Could you check a few things on this model? Use its own coordinates, in mm. A direction names the side the tool comes from. Coordinates: 2 decimals unless noted, no trailing zeros. Order: outer loops, then holes, each group sorted by start corner. A loop starts at its lowest first (then second) coordinate and runs counter-clockwise, first axis right, second up. Notation, with made-up numbers: (47.5, 44) - (86.5, 44) arc R14 cw to (86.5, 51) - close; hole circle Ø11 at (89.5, 71.25). An arc over 180 degrees is marked (long way). Answer as a JSON object with one key per item and string values. Group by question number.
(1) Imagine slicing it at D-D, the plane y = 19. Write out the boundary of the cut face in (x, z), and give its area (3 significant figures).
(2) Will these pins go through, and if not, where does the flat tip stop? P1, Ø8, axis at x = 50, y = -1.5, coming from the -Z side; P2, Ø3, axis at x = 42.5, y = 0, coming from the +Z side; P3, Ø1.5, axis at x = 49.5, z = 2, coming from the +Y side; P4, Ø1.5, axis at x = 49.5, z = 2, coming from the -Y side.
(3) We'd pull the mould along X, two halves only. Please class faces 3 (the flat face through (56.383, 0, 1)), 4 (the flat face through (50, -19.95, 1)), 5 (the cylindrical face through (31.8, -30.8, 1.5)): pulls with the +X half, pulls with the -X half, needs draft (parallel to the pull), parting line crosses it, or undercut.
(4) Imagine slicing it at A-A, the plane y = 0. Write out the boundary of the cut face in (x, z), and give its area (3 significant figures).
(5) Imagine slicing it at B-B, the plane x = 42.5. Write out the boundary of the cut face in (y, z), and give its area (3 significant figures).
(6) Which directions (+Z, -Z, +X, -X, +Y, -Y) give clear straight access to the entire face, cutting with the end or side of a thin tool? Please do faces 1 (the flat face through (50, 19.95, 1)), 2 (the flat face through (37, 1, 3)).
(7) Imagine slicing it at C-C, the plane z = 2.15. Write out the boundary of the cut face in (x, y) (3 decimals), and give its area (3 significant figures).
(8) Please list where these lines run through material, in increasing order: probe 1 along Y at (x, z) = (30, 1.65); probe 2 along Y at (x, z) = (42.5, 2.4); probe 3 along Y at (x, z) = (53, 1.95).
from build123d import *

# Parameters (mm, degrees)
SKETCH_1_R          = 47.75
SKETCH_1_R_2        = 32.5
SKETCH_1_R_3        = 1.9
EXTRUDE_1_DEPTH     = 3
SKETCH_2_R          = 1.9
CUT_EXTRUDE_1_DEPTH = 3
EXTRUDE_2_DEPTH     = 3
FILLET_1_R          = 3
FILLET_2_R          = 6


with BuildPart() as part:
    # 草图1 → 凸台-拉伸1 (new body)
    with BuildSketch(Plane.XY):
        Circle(SKETCH_1_R)
        Circle(SKETCH_1_R_2, mode=Mode.SUBTRACT)
        with Locations((0, 42.5)):
            Circle(SKETCH_1_R_3, mode=Mode.SUBTRACT)
        with Locations((30.0520382, 30.0520382)):
            Circle(SKETCH_1_R_3, mode=Mode.SUBTRACT)
        with Locations((42.5, 0)):
            Circle(SKETCH_1_R_3, mode=Mode.SUBTRACT)
        with Locations((30.0520382, -30.0520382)):
            Circle(SKETCH_1_R_3, mode=Mode.SUBTRACT)
        with Locations((0, -42.5)):
            Circle(SKETCH_1_R_3, mode=Mode.SUBTRACT)
        with Locations((-30.0520382, -30.0520382)):
            Circle(SKETCH_1_R_3, mode=Mode.SUBTRACT)
        with Locations((-42.5, 0)):
            Circle(SKETCH_1_R_3, mode=Mode.SUBTRACT)
        with Locations((-30.0520382, 30.0520382)):
            Circle(SKETCH_1_R_3, mode=Mode.SUBTRACT)
    extrude(amount=EXTRUDE_1_DEPTH)

    # 草图2 → 切除-拉伸1 (cut)
    # profile 1 of 2: a face of its own
    with BuildSketch(Plane(origin=(0, 0, 0), x_dir=(-1, 0, 0), z_dir=(0, 0, -1))):
        with BuildLine():
            ThreePointArc((40.6, 0), (42.5, 1.9), (44.4, 0))
            Line((44.4, 0), (47.75, 0))
            ThreePointArc((47.75, 0), (19.569412493, 43.555718278), (-31.709710772, 35.700934761))
            ThreePointArc((-31.709710772, 35.700934761), (-23.521159741, 36.955232453), (-19.021118385, 30))
            ThreePointArc((-19.021118385, 30), (-19.69088588, 26.875041473), (-21.582525806, 24.29906541))
            ThreePointArc((-21.582525806, 24.29906541), (13.319495322, 29.645253319), (32.5, 0))
            Line((32.5, 0), (40.6, 0))
        make_face()
        with Locations((0, 42.5)):
            Circle(SKETCH_2_R, mode=Mode.SUBTRACT)
        with Locations((30.0520382, 30.0520382)):
            Circle(SKETCH_2_R, mode=Mode.SUBTRACT)
    # profile 2 of 2: a face of its own
    with BuildSketch(Plane(origin=(0, 0, 0), x_dir=(-1, 0, 0), z_dir=(0, 0, -1))):
        with BuildLine():
            Line((47.75, 0), (44.4, 0))
            ThreePointArc((44.4, 0), (42.5, -1.9), (40.6, 0))
            Line((40.6, 0), (32.5, 0))
            ThreePointArc((32.5, 0), (13.319495418, -29.645253276), (-21.582525651, -24.299065549))
            ThreePointArc((-21.582525651, -24.299065549), (-19.690885837, -26.875041568), (-19.021118385, -30))
            ThreePointArc((-19.021118385, -30), (-23.521159897, -36.955232523), (-31.709711027, -35.700934534))
            ThreePointArc((-31.709711027, -35.700934534), (19.569412338, -43.555718347), (47.75, 0))
        make_face()
        with Locations((0, -42.5)):
            Circle(SKETCH_2_R, mode=Mode.SUBTRACT)
        with Locations((30.0520382, -30.0520382)):
            Circle(SKETCH_2_R, mode=Mode.SUBTRACT)
    extrude(amount=-CUT_EXTRUDE_1_DEPTH, mode=Mode.SUBTRACT)

    # 草图3 → 凸台-拉伸2 (add)
    with BuildSketch(Plane(origin=(0, 0, 0), x_dir=(-1, 0, 0), z_dir=(0, 0, -1))):
        with BuildLine():
            Line((-43.382715452, 19.95), (-56.382715452, 19.95))
            Line((-56.382715452, 19.95), (-56.382715452, 0))
            Line((-56.382715452, 0), (-47.75, 0))
            ThreePointArc((-47.75, 0), (-46.645402575, 10.211215333), (-43.382715452, 19.95))
        make_face()
        with BuildLine():
            Line((-47.75, 0), (-56.382715452, 0))
            Line((-56.382715452, 0), (-56.382715452, -19.95))
            Line((-56.382715452, -19.95), (-43.382715452, -19.95))
            ThreePointArc((-43.382715452, -19.95), (-46.645402575, -10.211215333), (-47.75, 0))
        make_face()
    extrude(amount=-EXTRUDE_2_DEPTH)

    # 圆角1
    fillet_1_edges = [part.edges().sort_by_distance(p)[0] for p in [
        (56.382715452, -19.95, 1.5),
        (56.382715452, 19.95, 1.5),
    ]]
    fillet(fillet_1_edges, radius=FILLET_1_R)

    # 圆角2
    fillet_2_edges = [part.edges().sort_by_distance(p)[0] for p in [
        (43.382715452, 19.95, 1.5),
        (43.382715452, -19.95, 1.5),
    ]]
    fillet(fillet_2_edges, radius=FILLET_2_R)


solid = part.part
Result set:
{
 "1": {"outline": "(26.37, 0) - (55.57, 0) - (55.57, 3) - (26.37, 3) - close", "area": "87.6 mm^2"},
 "2": {"P1": "stops at z = 0", "P2": "passes through", "P3": "stops at y = 19.95", "P4": "stops at y = -19.95"},
 "3": {"face 3": "pulls with the +X half", "face 4": "needs draft", "face 5": "undercut"},
 "4": {"outline": "(32.5, 0) - (40.6, 0) - (40.6, 3) - (32.5, 3) - close; (44.4, 0) - (56.38, 0) - (56.38, 3) - (44.4, 3) - close", "area": "60.2 mm^2"},
 "5": {"outline": "(-22.06, 0) - (-1.9, 0) - (-1.9, 3) - (-22.06, 3) - close; (1.9, 0) - (22.06, 0) - (22.06, 3) - (1.9, 3) - close", "area": "121 mm^2"},
 "6": {"face 1": "+Z, -Z, +X, +Y", "face 2": "+Z, +X, -X, +Y, -Y"},
 "7": {"outline": "(21.583, -24.299) arc R7.625 ccw to (31.71, -35.701) arc R47.75 ccw to (41.816, -23.053) arc R6 cw to (47.071, -19.95) - (53.383, -19.95) arc R3 ccw to (56.383, -16.95) - (56.383, 16.95) arc R3 ccw to (53.383, 19.95) - (47.071, 19.95) arc R6 cw to (41.816, 23.053) arc R47.75 ccw to (31.71, 35.701) arc R7.625 ccw to (21.583, 24.299) arc R32.5 cw to start; hole circle Ø3.8 at (30.052, -30.052); hole circle Ø3.8 at (30.052, 30.052); hole circle Ø3.8 at (42.5, 0)", "area": "1,580 mm^2"},
 "8": {"probe 1": "y = -36.85 to -31.95, -28.15 to -12.5, 12.5 to 28.15, 31.95 to 36.85", "probe 2": "y = -22.06 to -1.9, 1.9 to 22.06", "probe 3": "y = -19.95 to 19.95"}
}
